Verification items for the finished model (mm, model axes). A direction names the side the tool comes from. Give positions to 0.01 mm unless a question says otherwise; leave off trailing zeros. Write each loop counter-clockwise with the first axis right and the second up, starting at its lowest first coordinate (ties: lowest second). Pieces come first, ordered by that corner, then holes. Notation, with made-up numbers: M -35,20 L -2,20 A27 cw -2,54 Z; hole C 17,41 d2. An arc over 180 degrees is marked long. Write item = value, one per line.
from build123d import *

# Parameters (mm, degrees)
SKETCH_1_R               = 26
EXTRUDE_1_DEPTH          = 2
EXTRUDE_1_2_DEPTH        = 2
EXTRUDE_1_3_DEPTH        = 2
EXTRUDE_START            = 4
SKETCH_2_R               = 10
EXTRUDE_2_DEPTH          = 4
SKETCH_3_R               = 1.5
CUT_EXTRUDE_1_DEPTH      = 4
PATTERN_CIRCULAR_2_COUNT = 2
PATTERN_CIRCULAR_2_ANGLE = 100
F_2_THE_OTHER_WAY_COUNT  = 2
F_2_THE_OTHER_WAY_ANGLE  = 100
SKETCH_5_R               = 5
CUT_EXTRUDE_2_DEPTH      = 10
SKETCH_7_R               = 10
CUT_EXTRUDE_3_DEPTH      = 10


with BuildPart() as part:
    # Sketch 1 → Extrude 1 (new body)
    with BuildSketch(Plane(origin=(0, 0, 0), x_dir=(1, 0, 0), z_dir=(0, 1, 0))):
        with Locations(Location((0, 40, 0), (0, 0, 270))):
            Circle(SKETCH_1_R)
    extrude(amount=EXTRUDE_1_DEPTH)



with BuildPart() as body_2:
    # Sketch 1 → Extrude 1 2 (new body)
    with BuildSketch(Plane(origin=(0, 0, 0), x_dir=(1, 0, 0), z_dir=(0, 1, 0))):
        with Locations(Location((39.39231012, -6.945927107, 0), (0, 0, 270))):
            Circle(SKETCH_1_R)
    extrude(amount=EXTRUDE_1_2_DEPTH)


with BuildPart() as body_3:
    # Sketch 1 → Extrude 1 3 (new body)
    with BuildSketch(Plane(origin=(0, 0, 0), x_dir=(1, 0, 0), z_dir=(0, 1, 0))):
        with Locations(Location((-39.39231012, -6.945927107, 0), (0, 0, 270))):
            Circle(SKETCH_1_R)
    extrude(amount=EXTRUDE_1_3_DEPTH)


with BuildPart() as part_1:
    add(part.part)

    add(body_2.part)  # Extrude 2 merges body 2

    add(body_3.part)  # Extrude 2 merges body 3
    # Sketch 2 → Extrude 2 (add)
    with BuildSketch(Plane.XZ.offset(EXTRUDE_START)):
        with BuildLine():
            Line((-39.39231012, 32.945927107), (39.39231012, 32.945927107))
            ThreePointArc((39.39231012, 32.945927107), (62.956312583, 17.934001912), (59.309465642, -9.766550745))
            Line((59.309465642, -9.766550745), (19.917155521, -56.712477852))
            ThreePointArc((19.917155521, -56.712477852), (0, -66), (-19.917155521, -56.712477852))
            Line((-19.917155521, -56.712477852), (-59.309465642, -9.766550745))
            ThreePointArc((-59.309465642, -9.766550745), (-62.956312583, 17.934001912), (-39.39231012, 32.945927107))
        make_face()
        with Locations(Location((0, 0, 0), (0, 0, 270))):
            Circle(SKETCH_2_R, mode=Mode.SUBTRACT)
    extrude(amount=-EXTRUDE_2_DEPTH)

    # Sketch 3 → Cut-Extrude 1 (cut)
    with BuildSketch(Plane(origin=(0, 0, 0), x_dir=(1, 0, 0), z_dir=(0, 1, 0))):
        with Locations(Location((12.374368671, 12.374368671, 0), (0, 0, 270))):
            Circle(SKETCH_3_R)
        with Locations(Location((-12.374368671, 12.374368671, 0), (0, 0, 90))):
            Circle(SKETCH_3_R)
        with Locations(Location((-12.374368671, -12.374368671, 0), (0, 0, 270))):
            Circle(SKETCH_3_R)
        with Locations(Location((12.374368671, -12.374368671, 0), (0, 0, 90))):
            Circle(SKETCH_3_R)
        with Locations(Location((0, -17.5, 0), (0, 0, 270))):
            Circle(SKETCH_3_R)
    extrude(amount=-CUT_EXTRUDE_1_DEPTH, mode=Mode.SUBTRACT)

    # Sketch 4 → Revolve 1 (revolve)
    with BuildSketch(Plane(origin=(0, 0, 0), x_dir=(0, 0, -1), z_dir=(1, 0, 0)), mode=Mode.PRIVATE) as revolve_1_sk:
        Polygon((68.570552361, 9.72740661), (67.070552361, 9.72740661), (65, 2), (66, 2), (66, 0), align=None)
    revolve_1 = revolve(revolve_1_sk.sketch.rotate(Axis((0, 2, -40), (0, 1, 0)), 180), axis=Axis((0, 2, -40), (0, 1, 0)))

    # Pattern Circular 2: Revolve 1 ×2 about axis
    pattern_circular_2_axis = Axis((0, -6.257104181, 0), (0, 1, 0))
    for i in range(1, PATTERN_CIRCULAR_2_COUNT):
        add(revolve_1.rotate(pattern_circular_2_axis, i * PATTERN_CIRCULAR_2_ANGLE / (PATTERN_CIRCULAR_2_COUNT - 1)))

    # 2 the other way: Revolve 1 ×2 about axis
    f_2_the_other_way_axis = Axis((0, -6.257104181, 0), (0, -1, 0))
    for i in range(1, F_2_THE_OTHER_WAY_COUNT):
        add(revolve_1.rotate(f_2_the_other_way_axis, i * F_2_THE_OTHER_WAY_ANGLE / (F_2_THE_OTHER_WAY_COUNT - 1)))

    # Sketch 5 → Cut-Extrude 2 (cut)
    with BuildSketch(Plane(origin=(0, 0, 0), x_dir=(1, 0, 0), z_dir=(0, 1, 0))):
        with Locations((12.374368671, -12.374368671)):
            Circle(SKETCH_5_R)
        with Locations((-12.374368671, -12.374368671)):
            Circle(SKETCH_5_R)
    extrude(amount=CUT_EXTRUDE_2_DEPTH, mode=Mode.SUBTRACT)

    # Sketch 7 → Cut-Extrude 3 (cut)
    with BuildSketch(Plane(origin=(0, 2, 0), x_dir=(1, 0, 0), z_dir=(0, 1, 0))):
        with Locations(Location((0, 40, 0), (0, 0, 270))):
            Circle(SKETCH_7_R)
    extrude(amount=-CUT_EXTRUDE_3_DEPTH, mode=Mode.SUBTRACT)


solid = part_1.part
1) Draft check along Z on faces 4 (the conical face through (-64.804, 0.609, 0.732)), 5 (the cylindrical face through (0, -2, -66)), 6 (the flat face through (-1, -2, 32.946)). Enter one of: +Z half, -Z half, draft (parallel to the pull), parting line (faces both ways), or undercut.
From the geometry:
face_4 = undercut
face_5 = -Z half
face_6 = +Z half
2) Cross-section at A-A on y = 7.5. Record the boundary of the cut face in (x, z).
From the geometry:
outline = C 0,-40 d55.96; M -14.8,16.75 A5 cw -13.39,17.27 A27.98 ccw long -11.42,7.47 A5 cw -12.92,7.4 A26.47 cw long Z; M 11.42,7.47 A27.98 ccw long 13.39,17.27 A5 cw 14.8,16.75 A26.47 cw long 12.92,7.4 A5 cw Z; hole C 0,-40 d52.95
3) Cross-section at C-C on z = -40. Record the boundary of the cut face in (x, y).
From the geometry:
outline = M -33.94,-4 L -10,-4 L -10,2 L -25,2 L -27.07,9.73 L -28.57,9.73 L -26,0 L -33.94,0 Z; M 10,-4 L 33.94,-4 L 33.94,0 L 26,0 L 28.57,9.73 L 27.07,9.73 L 25,2 L 10,2 Z
4) Material ranges on probe 1 along Z at (x, y) = (19, 3.25); probe 2 along Z at (x, y) = (-19, 5.25); probe 3 along Y at (x, z) = (38.5, -27.5), recorded low to high. Write a range as from..to.
From the geometry:
probe_1 = -58.98..-56.76, -23.24..-21.02, -10.53..-8.09, 21.98..24.43
probe_2 = -59.72..-57.56, -22.44..-20.28, -11.34..-8.97, 22.87..25.23
probe_3 = -4..0
5) Cross-section at B-B on x = 0. Record the boundary of the cut face in (y, z), plus the area to 3 significant figures.
From the geometry:
outline = M -4,-66 L 0,-66 L 9.73,-68.57 L 9.73,-67.07 L 2,-65 L 2,-50 L -4,-50 Z; M -4,-30 L 2,-30 L 2,-15 L 9.73,-12.93 L 9.73,-11.43 L 0,-14 L 0,-10 L -4,-10 Z; M -4,10 L 0,10 L 0,16 L -4,16 Z; M -4,19 L 0,19 L 0,32.95 L -4,32.95 Z
area = 312 mm^2
6) Depth check by flat-ended pin: P1, Ø4.5, axis at x = 11.5, y = -3, coming from the +Z side; P2, Ø6, axis at x = -12.37, z = 12.37, coming from the +Y side; P3, Ø4, axis at x = 53.5, y = -2.5, coming from the +Z side; P4, Ø2.5, axis at x = -12.37, z = 12.37, coming from the +Y side. Enter the tip coordinate at first touch or a pass-through.
From the geometry:
P1 = 32.95
P2 = 0
P3 = 29.95
P4 = through
7) Tool access check on faces 1 (the cylindrical face through (62.779, -2.028, 18.307)), 2 (the flat face through (40, 2, 7)), 3 (the conical face through (65.232, 0.609, 2.862)). Record the directions out of +Z, -Z, +X, -X, +Y, -Y that give a thin tool (end or side, any length) a straight path to the whole face; none if there is none.
From the geometry:
face_1 = +X, -Y
face_2 = +Y
face_3 = none
